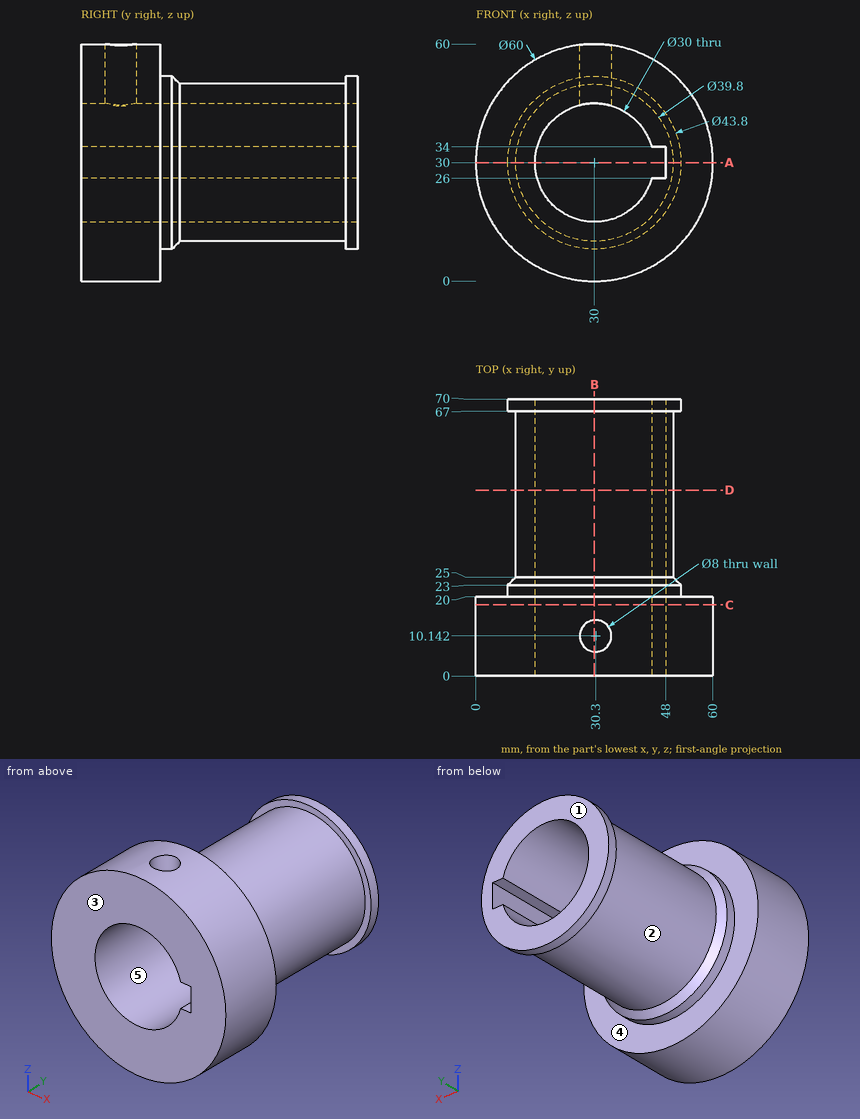
Geometry: see drawing. Coordinates: mm, zero at the bounding-box minimum. A direction names the side the tool comes from. Round coordinates to 2 decimals unless told otherwise and drop trailing zeros. Loops run counter-clockwise (first coordinate to the right, second up) from the corner with the lowest first, then second, coordinate; pieces in that order, holes last. Notation, with made-up numbers: (57.5, 8) - (116.5, 8) arc R23 ccw to (116.5, 18) - close; hole circle Ø5 at (-32, 61). An arc over 180 degrees is marked (long way). One line per item, written item: value. Start each with the question number.
(1) Section B-B, the plane x = 30. Return loops of the section in (y, z).
(2) Draft query along Y for the marked faces 1, 2 and 3. Return one class per face: +Y half, -Y half, draft (parallel to the pull), parting line (faces both ways), or undercut.
(3) Section C-C, the plane y = 18. Return loops of the section in (x, z), plus the area to 4 significant figures.
(4) Access query for the marked faces 4 and 5. Directions: +Z, -Z, +X, -X, +Y, -Y. A direction counts if a zero-diameter tool reaches every point of the face in a straight line with its end or side. Return the directions, or none.
(5) Section D-D, the plane y = 47. Return loops of the section in (x, z).
(6) Contact query for flat-ended pins moving along their axis: P1, Ø3, axis at x = 51, y = 11, coming from the -Z side; P2, Ø4, axis at x = 45.5, y = 45, coming from the -Z side; P3, Ø1, axis at y = 43, z = 27, coming from the +X side; P4, Ø10.5, axis at x = 30.3, y = 10.14, coming from the +Z side. Output: stop coordinate, or through.
(7) Ray query, line 1 (Z direction, x = 30, y = 40); line 2 (Y direction, x = 42.5, z = 53); line 3 (X direction, y = 10, z = 45). Return the intervals inside material, ascending. Write a range as [from, to].
(8) Section A-A, the plane z = 30. Return loops of the section in (x, y).
Results below:
1. outline: (0, 0) - (20, 0) - (20, 8.1) - (23, 8.1) - (25, 10.1) - (67, 10.1) - (67, 8.1) - (70, 8.1) - (70, 15) - (0, 15) - close; (0, 45) - (6.15, 45) - (6.15, 60) - (0, 60) - close; (14.13, 45) - (70, 45) - (70, 51.9) - (67, 51.9) - (67, 49.9) - (25, 49.9) - (23, 51.9) - (20, 51.9) - (20, 60) - (14.13, 60) - close
2. face 1: +Y half
2. face 2: undercut
2. face 3: -Y half
3. outline: circle Ø60 at (30, 30); hole (44.46, 26) - (48, 26) - (48, 34) - (44.46, 34) arc R15 ccw (long way) to start
3. area: 2,095 mm^2
4. face 4: +Y
4. face 5: +Y, -Y
5. outline: circle Ø39.8 at (30, 30); hole (44.46, 26) - (48, 26) - (48, 34) - (44.46, 34) arc R15 ccw (long way) to start
6. P1: z = 7.2
6. P2: z = 15.38
6. P3: x = 49.74
6. P4: z = 60
7. line 1: [10.1, 15], [45, 49.9]
7. line 2: [0, 20]
7. line 3: [4.02, 26.3], [34.3, 55.98]
8. outline: (0, 0) - (15, 0) - (15, 70) - (8.1, 70) - (8.1, 67) - (10.1, 67) - (10.1, 25) - (8.1, 23) - (8.1, 20) - (0, 20) - close; (48, 0) - (60, 0) - (60, 20) - (51.9, 20) - (51.9, 23) - (49.9, 25) - (49.9, 67) - (51.9, 67) - (51.9, 70) - (48, 70) - close
